from build123d import *
from OCP.BRepFilletAPI import BRepFilletAPI_MakeChamfer

# Parameters (mm, degrees)
DOWELSUPPORT_DEPTH       = 1.905
DOWELSUPPORT_DEPTH_BACK  = 1.27
SKETCH3_R                = 3.81
SKETCH5_W                = 9.525
SKETCH5_H                = 19.05
SLIDERDOWELSUPPORT_DEPTH = 1.27
STRINGDOWELSUPPORT_DEPTH = 1.27
SKETCH9_W                = 6.35
SKETCH9_H                = 3
TABSUPPORT_DEPTH         = 1.27
INTERSUPPORT_DEPTH       = 1.27
DOWELHOLES_DEPTH         = 30.584731096
DOWELHOLES_DEPTH_BACK    = 30.584731096
SKETCH11_R               = 1.600000102
BOSS_EXTRUDE1_START      = -1.27
SKETCH11_2_R             = 1.600000102
BOSS_EXTRUDE1_DEPTH      = 0.254
SKETCH14_W               = 6.35
SKETCH14_H               = 3
TABBASE_DEPTH            = 1.27
SKETCH15_W               = 6.35
SKETCH15_H               = 3
TABDRAFT_DEPTH           = 1.73
TABDRAFT_DRAFT           = 5
TABDRAFT_PROFILE_2_DEPTH = 1.73
TABDRAFT_PROFILE_2_DRAFT = 5
CHAMFER1_SIZE            = 2.54
CUT_EXTRUDE1_DEPTH       = 3
CHAMFER2_SIZE            = 0.508
CHAMFER2_SIZE2           = 1.016


with BuildPart() as part:
    # Sketch3 → DowelSupport (new, two sides: drawn at the far end of the back side and taken through both)
    with BuildSketch(Plane(origin=(0, 0, 0), x_dir=(0, 0, -1), z_dir=(1, 0, 0)).offset(-DOWELSUPPORT_DEPTH_BACK)):
        with Locations((-3.175, 20.88375)):
            Circle(SKETCH3_R)
    extrude(amount=DOWELSUPPORT_DEPTH + DOWELSUPPORT_DEPTH_BACK)



with BuildPart() as body_2:
    # Sketch5 → SliderDowelSupport (new, symmetric)
    with BuildSketch(Plane(origin=(0, 0, 0), x_dir=(0, 0, -1), z_dir=(1, 0, 0))):
        with Locations((-1.5875, 0)):
            Rectangle(SKETCH5_W, SKETCH5_H)
    extrude(amount=SLIDERDOWELSUPPORT_DEPTH, both=True)


with BuildPart() as body_3:
    # Sketch8 → StringDowelSupport (new, symmetric)
    with BuildSketch(Plane(origin=(0, 0, 0), x_dir=(0, 0, -1), z_dir=(1, 0, 0))):
        with BuildLine():
            Line((4.6355, 24.892), (8.0645, 24.892))
            ThreePointArc((8.0645, 24.892), (10.6045, 22.352), (8.0645, 19.812))
            Line((8.0645, 19.812), (4.6355, 19.812))
            ThreePointArc((4.6355, 19.812), (2.0955, 22.352), (4.6355, 24.892))
        make_face()
    extrude(amount=STRINGDOWELSUPPORT_DEPTH, both=True)


with BuildPart() as part_1:
    add(part.part)

    add(body_3.part)  # TabSupport merges body 3
    # Sketch9 → TabSupport (add, symmetric)
    with BuildSketch(Plane(origin=(0, 0, 0), x_dir=(0, 0, -1), z_dir=(1, 0, 0))):
        with Locations((0, 21.59)):
            Rectangle(SKETCH9_W, SKETCH9_H)
        with Locations((12.7, 21.59)):
            Rectangle(SKETCH9_W, SKETCH9_H)
    extrude(amount=TABSUPPORT_DEPTH, both=True)


    add(body_2.part)  # InterSupport merges body 2
    # Sketch10 → InterSupport (add, symmetric)
    with BuildSketch(Plane(origin=(0, 0, 0), x_dir=(0, 0, -1), z_dir=(1, 0, 0))):
        Polygon((-6.35, 9.525), (-5.711088789, 21.024652996), (-3.644260291, 23.380026182), (4.166239709, 24.848276182), (8.657140431, 24.821894192), (15.875, 23.09), (15.875, 20.09), (3.175, 3.175), (3.175, 9.525), align=None)
    extrude(amount=INTERSUPPORT_DEPTH, both=True)

    # Sketch11 → DowelHoles (cut, two sides: drawn at the far end of the back side and taken through both)
    with BuildSketch(Plane(origin=(0, 0, 0), x_dir=(0, 0, -1), z_dir=(1, 0, 0)).offset(-DOWELHOLES_DEPTH_BACK)):
        with Locations((-3.175, 20.88375)):
            Circle(SKETCH11_R)
        with BuildLine():
            Line((6.04239599, 21.59), (6.65760401, 21.59))
            ThreePointArc((6.65760401, 21.59), (9.664500102, 22.352), (6.65760401, 23.114))
            Line((6.65760401, 23.114), (6.04239599, 23.114))
            ThreePointArc((6.04239599, 23.114), (3.035499898, 22.352), (6.04239599, 21.59))
        make_face()
    extrude(amount=DOWELHOLES_DEPTH + DOWELHOLES_DEPTH_BACK, mode=Mode.SUBTRACT)

    # Sketch11<2> → Boss-Extrude1 (add)
    with BuildSketch(Plane(origin=(0, 0, 0), x_dir=(0, 0, -1), z_dir=(1, 0, 0)).offset(BOSS_EXTRUDE1_START)):
        with BuildLine():
            Line((6.04239599, 21.59), (6.65760401, 21.59))
            ThreePointArc((6.65760401, 21.59), (9.664500102, 22.352), (6.65760401, 23.114))
            Line((6.65760401, 23.114), (6.04239599, 23.114))
            ThreePointArc((6.04239599, 23.114), (3.035499898, 22.352), (6.04239599, 21.59))
        make_face()
        with Locations((-3.175, 20.88375)):
            Circle(SKETCH11_2_R)
    extrude(amount=BOSS_EXTRUDE1_DEPTH)

    # Sketch14 → TabBase (add)
    with BuildSketch(Plane.ZY.offset(1.27)):
        with Locations((-12.7, 21.59)):
            Rectangle(SKETCH14_W, SKETCH14_H)
        with Locations((0, 21.59)):
            Rectangle(SKETCH14_W, SKETCH14_H)
    extrude(amount=TABBASE_DEPTH)


with BuildPart() as tabdraft_tool:
    # Sketch15 → TabDraft (with draft: the straight prism first)
    with BuildSketch(Plane.ZY.offset(2.54)):
        with Locations((0, 21.59)):
            Rectangle(SKETCH15_W, SKETCH15_H)
    extrude(amount=TABDRAFT_DEPTH)
    # TabDraft: the draft: its side faces are tilted about the plane it starts from
    tabdraft_sides = [tabdraft_tool.faces().sort_by_distance(p)[0] for p in [
        (-3.405, 21.59, -3.175),
        (-3.405, 20.09, 0),
        (-3.405, 21.59, 3.175),
        (-3.405, 23.09, 0),
    ]]
    draft(tabdraft_sides, Plane.ZY.offset(2.54), TABDRAFT_DRAFT)


with BuildPart() as part_2:
    add(part_1.part)

    # TabDraft: add tabdraft_tool
    add(tabdraft_tool.part)


with BuildPart() as tabdraft_profile_2_tool:
    # Sketch15 → TabDraft profile 2 (with draft: the straight prism first)
    with BuildSketch(Plane.ZY.offset(2.54)):
        with Locations((-12.7, 21.59)):
            Rectangle(SKETCH15_W, SKETCH15_H)
    extrude(amount=TABDRAFT_PROFILE_2_DEPTH)
    # TabDraft profile 2: the draft: its side faces are tilted about the plane it starts from
    tabdraft_profile_2_sides = [tabdraft_profile_2_tool.faces().sort_by_distance(p)[0] for p in [
        (-3.405, 21.59, -15.875),
        (-3.405, 20.09, -12.7),
        (-3.405, 21.59, -9.525),
        (-3.405, 23.09, -12.7),
    ]]
    draft(tabdraft_profile_2_sides, Plane.ZY.offset(2.54), TABDRAFT_PROFILE_2_DRAFT)


with BuildPart() as part_3:
    add(part_2.part)

    # TabDraft profile 2: add tabdraft_profile_2_tool
    add(tabdraft_profile_2_tool.part)

    # Chamfer1
    chamfer1_edges = [part_3.edges().sort_by_distance(p)[0] for p in [
        (1.27, 11.6325, -9.525),
    ]]
    chamfer(chamfer1_edges, length=CHAMFER1_SIZE - 0.0001)  # a hair under: the kernel refuses the full size

    # Mirror1: part across plane


with BuildPart() as part_4:
    add(part_3.part)
    add(part_3.part.mirror(Plane.ZX))

    # Sketch16 → Cut-Extrude1 (cut)
    with BuildSketch(Plane.XY.offset(6.35)):
        Polygon((-1.27, -4.006469684), (1.27, -2.54), (1.27, 2.54), (-1.27, 4.006469684), align=None)
    extrude(amount=-CUT_EXTRUDE1_DEPTH, mode=Mode.SUBTRACT)

    # Chamfer2: one chamfer whose edges measure the first distance from different faces: ONE call of the kernel's chamfer builder (chamfer() names one face for all edges)
    chamfer2_edges_1 = [part_4.edges().sort_by_distance(p)[0] for p in [
        (0, -3.273234842, 6.35),
    ]]
    chamfer2_side_1 = [part_4.faces().sort_by_distance(p)[0] for p in [
        (0.049650417, -6.38478458, 6.35),
    ]]
    chamfer2_edges_2 = [part_4.edges().sort_by_distance(p)[0] for p in [
        (0, 3.273234842, 6.35),
    ]]
    chamfer2_side_2 = [part_4.faces().sort_by_distance(p)[0] for p in [
        (0.049650417, 6.38478458, 6.35),
    ]]
    chamfer2 = BRepFilletAPI_MakeChamfer(part_4.part.solid().wrapped)
    for e in chamfer2_edges_1:
        chamfer2.Add(CHAMFER2_SIZE, CHAMFER2_SIZE2, e.wrapped, chamfer2_side_1[0].wrapped)  # the first distance lies on this face
    for e in chamfer2_edges_2:
        chamfer2.Add(CHAMFER2_SIZE, CHAMFER2_SIZE2, e.wrapped, chamfer2_side_2[0].wrapped)  # the first distance lies on this face
    add(Compound.cast(chamfer2.Shape()), mode=Mode.REPLACE)


solid = part_4.part
Input: part model. Units: mm. Frame: model coordinates. A direction names the side the tool comes from. Coordinates: 2 decimals unless noted, no trailing zeros. Write each loop counter-clockwise with the first axis right and the second up, starting at its lowest first coordinate (ties: lowest second). Pieces come first, ordered by that corner, then holes. Notation, with made-up numbers: M 75.25,-1.75 L 113.25,-1.75 A17 ccw 113.25,19.25 Z; hole C -9,24 d3. An arc over 180 degrees is marked long. Answer as a JSON object with one key per item and string values. Group by question number.
(1) Mould query, pull axis Y, two halves, no side actions, for faces 5 (the face through (0.018, 23.968, -12.216)), 6 (the face through (-3.4, -21.6, 3.1)), 7 (the face through (0.018, -13.796, 6.113)). Classes: pulls with the +Y half, pulls with the -Y half, needs draft (parallel to the pull), parting line crosses it, or undercut.
(2) Ray query, line 1 along Y through (x, z) = (-1.75, -0.25); line 2 along X through (y, z) = (-14.5, -0.5); line 3 along Y through (x, z) = (1.5, 6). Return the intervals inside material, ascending. Write a range as [from, to].
(3) Set-up query: faces 1 (the face through (0, 0, 3.35)), 2 (the face through (-2, 23.09, 0)), 3 (the face through (0.02, -24.37, -1.62)), 4 (the face through (-2, 22, -9.525)). Return all of +Z, -Z, +X, -X, +Y, -Y with unobstructed straight access to the full face (end or side cutting, diameter ignored); none if empty.
(4) Section A-A on x = -3.5. Output: boundary loops of the cut face in (y, z), plus the area to 3 significant figures.
(5) Contact query for flat-ended pins moving along their axis: P1, Ø7, axis at y = 12, z = -4.5, coming from the -X side; P2, Ø1, axis at x = -2, z = -14, coming from the +Y side; P3, Ø1.5, axis at y = 12.5, z = -7, coming from the +X side; P4, Ø4, axis at y = 22.35, z = -8.06, coming from the -X side. Output: stop coordinate, or through.
Result set:
{
 "1": {"face 5": "pulls with the +Y half", "face 6": "needs draft", "face 7": "undercut"},
 "2": {"line 1": "y = [-23.09, -20.09], [20.09, 23.09]", "line 2": "x = [-1.27, 1.27]", "line 3": "y = [-23.44, -18.33], [18.33, 23.44]"},
 "3": {"face 1": "+Z, -X", "face 2": "+Z, -Z, -X, +Y", "face 3": "+X, -X, -Y", "face 4": "-X, +Y, -Y"},
 "4": {"outline": "M -23.01,-15.79 L -20.17,-15.79 L -20.17,-9.61 L -23.01,-9.61 Z; M -23.01,-3.09 L -20.17,-3.09 L -20.17,3.09 L -23.01,3.09 Z; M 20.17,-15.79 L 23.01,-15.79 L 23.01,-9.61 L 20.17,-9.61 Z; M 20.17,-3.09 L 23.01,-3.09 L 23.01,3.09 L 20.17,3.09 Z", "area": "70.0 mm2"},
 "5": {"P1": "stops at x = -1.27", "P2": "stops at y = 23.09", "P3": "stops at x = 1.27", "P4": "stops at x = -4.27"}
}
